Could you check a few things on this drawing? It's one solid part, dimensions in mm from its lowest x, y, z. Coordinates: 2 decimals unless noted, no trailing zeros. Write each loop counter-clockwise with the first axis right and the second up, starting at its lowest first coordinate (ties: lowest second). Pieces come first, ordered by that corner, then holes.
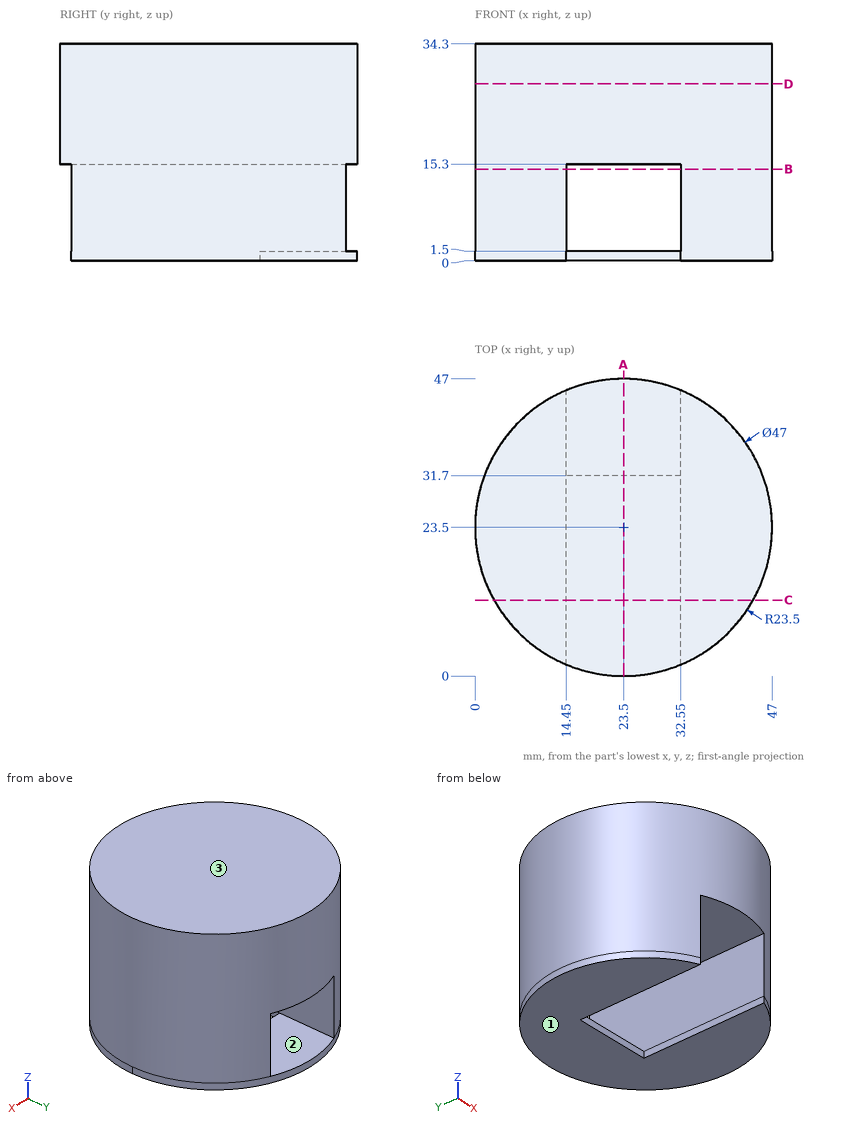
1) We'd pull the mould along Z, two halves only. Please class the marked faces 1, 2 and 3: pulls with the +Z half, pulls with the -Z half, needs draft (parallel to the pull), parting line crosses it, or undercut.
Values follow:
face 1: pulls with the -Z half
face 2: undercut
face 3: pulls with the +Z half
2) Will these pins go through, and if not, where does the flat tip stop? pin 1 (1.6 mm diameter, centred on y = 14, z = 1, fed in from +X); pin 2 (12 mm diameter, centred on y = 35.5, z = 3.5, fed in from +X); pin 3 (7 mm diameter, centred on y = 32.5, z = 10, fed in from +X).
Values follow:
pin 1: stops at x = 45.33
pin 2: stops at x = 46.22
pin 3: stops at x = 46.35
3) I need wall thicknesses on probe 1 along Z at (x, y) = (20.5, 42.5); probe 2 along X at (y, z) = (27.5, 8); probe 3 along Z at (x, y) = (27.5, 19). Which ranges of each line are inside material? Lowest first, please.
Values follow:
probe 1: z = 0 to 1.5, 15.3 to 34.3
probe 2: x = 0.34 to 14.45, 32.55 to 46.66
probe 3: z = 15.3 to 34.3
4) Imagine slicing it at D-D on z = 28. Please give me the cut outline in (x, y).
Values follow:
outline: circle Ø47 at (23.5, 23.5)
5) Imagine slicing it at C-C on y = 12. Please give me the cut outline in (x, z).
Values follow:
outline: (3.01, 0) - (14.45, 0) - (14.45, 15.3) - (32.55, 15.3) - (32.55, 0) - (43.99, 0) - (43.99, 34.3) - (3.01, 34.3) - close
6) Imagine slicing it at B-B on z = 14.5. Please give me the cut outline in (x, y), then the cut area to 3 significant figures.
Values follow:
outline: (14.45, 1.81) - (14.45, 45.19) arc R23.5 ccw to start; (32.55, 1.81) arc R23.5 ccw to (32.55, 45.19) - close
area: 906 mm2
7) Imagine slicing it at A-A on x = 23.5. Please give me the cut outline in (y, z).
Values follow:
outline: (0, 15.3) - (47, 15.3) - (47, 34.3) - (0, 34.3) - close; (31.7, 0) - (47, 0) - (47, 1.5) - (31.7, 1.5) - close
